Geometry check sheet. Reference: the model listing, model coordinates, mm. Round coordinates to 2 decimals unless told otherwise and drop trailing zeros. Order: outer loops, then holes, each group sorted by start corner. A loop starts at its lowest first (then second) coordinate and runs counter-clockwise, first axis right, second up.
(1) Gauge pin test, flat ends, axial feed: P1, Ø10, axis at y = 41, z = -158.5, coming from the -X side; P2, Ø6, axis at x = -13, y = 10.5, coming from the -Z side. Record the tip position at first contact, or that the pin passes through.
(2) Cross-section at B-B on y = 5. Enter the section's corners in (x, z).
(3) Thickness scan on L1, parallel to X at y = 67.5, z = -217; L2, parallel to Z at x = -23, y = 52.5; L3, parallel to Z at x = -36.5, y = 12. Record the ranges inside material, lowest first.
(4) Cross-section at A-A on z = -118.5. Enter the section's corners in (x, y) (3 decimals), and give its area (3 significant figures).
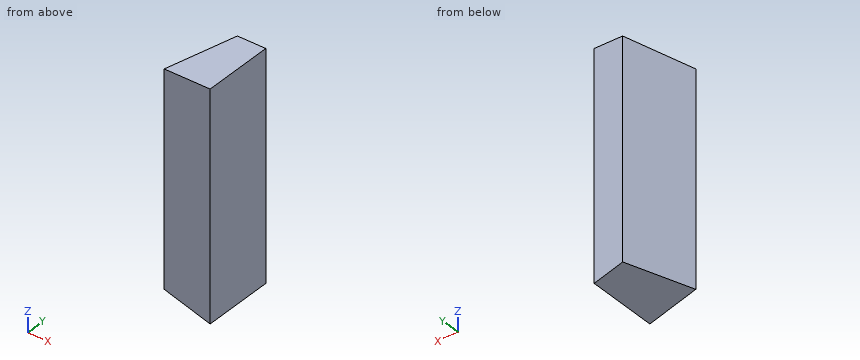
Autodesk Inventor part; units mm, degrees
ref_plane "Work Plane1" through (-8.9942, -7.112, -242.5521) normal (-0.2905, 0, -0.9569) x (0, 1, 0)
ref_plane "YZ Plane" through (0, 0, 0) normal (1, 0, 0) x (0, 1, 0)
ref_plane "XZ Plane" through (0, 0, 0) normal (0, 1, 0) x (-1, 0, 0)
sketch "Sketch1" plane through (0, 0, 0) normal (0, 0, 1) x (1, 0, 0)
  line L0 (-812.8, -3.937) -> (0, -3.937)
  line L1 (-30.988, 74.295) -> (-15.2847, 74.295)
  line L2 (0, -3.937) -> (-50.038, -3.937)
  line L3 (-50.038, -3.937) -> (-30.988, 74.295)
  line L4 (-30.988, 74.295) -> (0, 74.295)
  line L5 (0, 74.295) -> (0, -3.937)
  line L6 (-50.038, -7.112) -> (-50.038, -3.937)
  point P0 (0, 0)
ref_plane "Work Plane1" through (-8.9942, -7.112, -242.5521) normal (-0.2905, 0, -0.9569) x (0, 1, 0)
extrude "Extrusion1" add sketch "Sketch1" against normal up to surface surface through (-8.9942, -7.112, -242.5521) normal (-0.2905, 0, -0.9569)
properties part number "FrontBumperFillA"
Found:
1. P1: stops at x = -40.31
1. P2: stops at z = -242.25
2. outline: (-47.86, -230.75) - (0, -245.28) - (0, 0) - (-47.86, 0) - close
3. L1: x = -32.64 to 0
3. L2: z = -238.3 to 0
3. L3: z = -234.2 to 0
4. outline: (-50.038, -3.937) - (0, -3.937) - (0, 74.295) - (-30.988, 74.295) - close
4. area: 3,170 mm2
